Check sheet for the modelled part. Datum: model origin and axes. Units: mm. Round coordinates to 2 decimals unless told otherwise and drop trailing zeros. Write each loop counter-clockwise with the first axis right and the second up, starting at its lowest first coordinate (ties: lowest second). Pieces come first, ordered by that corner, then holes. Notation, with made-up numbers: (66, -1) -> (101, -1) arc R22 ccw to (101, 32) -> close; hole circle Ø9 at (35, 36). An arc over 180 degrees is marked (long way). Put each result on its own line as item: value. Start each with the question number.
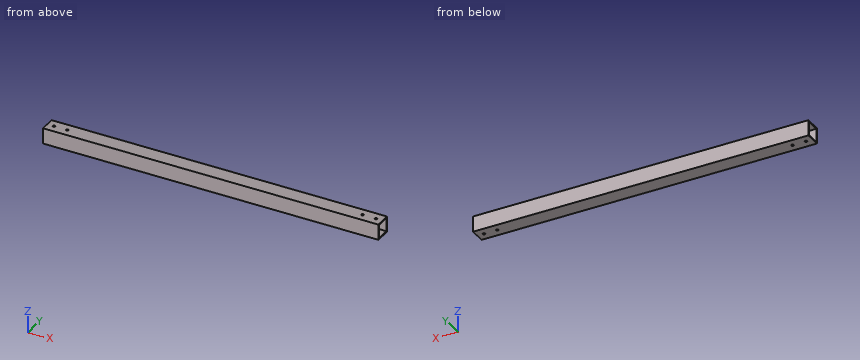
from build123d import *

# Parameters (mm, degrees)
SKETCH1_W               = 44.45
SKETCH1_H               = 44.45
SKETCH1_W_2             = 38.1
SKETCH1_H_2             = 38.1
BOSS_EXTRUDE1_DEPTH     = 954.786
F_1_4_CLEARANCE_HOLE1_D = 6.7564


with BuildPart() as part:
    # Sketch1 → Boss-Extrude1 (new body)
    with BuildSketch(Plane(origin=(0, 0, 0), x_dir=(0, 0, -1), z_dir=(1, 0, 0))):
        with Locations((22.225, 22.225)):
            Rectangle(SKETCH1_W, SKETCH1_H)
        with Locations((22.225, 22.225)):
            Rectangle(SKETCH1_W_2, SKETCH1_H_2, mode=Mode.SUBTRACT)
    extrude(amount=BOSS_EXTRUDE1_DEPTH)

    # 1/4 Clearance Hole1 (through all)
    with Locations(Plane.XY):
        with Locations((19.05, 22.225), (57.15, 22.225), (935.736, 22.225), (897.636, 22.225)):
            Hole(F_1_4_CLEARANCE_HOLE1_D / 2)


solid = part.part
1. Section check A-A, the plane z = -24. Enter the section's corners in (x, y) (3 decimals), then the cut area to 3 significant figures.
2. Gauge pin test, flat end, axial feed: P1, Ø5.5, axis at x = 935.736, y = 22.225, coming from the -Z side. Record the tip position at first contact, or that the pin passes through.
3. Section check B-B, the plane x = 199. Enter the section's corners in (y, z) (3 decimals), then the cut area to 3 significant figures.
4. Material ranges on L1, parallel to Y at x = 841, z = -23 (3 decimals); L2, parallel to Z at x = 173.5, y = 35.5 (3 decimals); L3, parallel to Y at x = 57.15, z = -43.6, recorded low to high. Write a range as [from, to].
Reply:
1. outline: (0, 0) -> (954.786, 0) -> (954.786, 3.175) -> (0, 3.175) -> close; (0, 41.275) -> (954.786, 41.275) -> (954.786, 44.45) -> (0, 44.45) -> close
1. area: 6,060 mm2
2. P1: passes through
3. outline: (0, -44.45) -> (44.45, -44.45) -> (44.45, 0) -> (0, 0) -> close; hole (3.175, -41.275) -> (41.275, -41.275) -> (41.275, -3.175) -> (3.175, -3.175) -> close
3. area: 524 mm2
4. L1: y = [0, 3.175], [41.275, 44.45]
4. L2: z = [-44.45, -41.275], [-3.175, 0]
4. L3: y = [0, 18.85], [25.6, 44.45]
